CAD build for the part. Positions are in the model's coordinates, mm. A direction names the side the tool comes from. Coordinates: 2 decimals unless noted, no trailing zeros. Order: outer loops, then holes, each group sorted by start corner. A loop starts at its lowest first (then second) coordinate and runs counter-clockwise, first axis right, second up. Notation, with made-up numbers: M 82,86 L 104,86 A14 ccw 104,106 Z; hole C 1,64.25 d3. An arc over 180 degrees is marked long. Write item = value, one per line.
from build123d import *

# Parameters (mm, degrees)
SALIENTE_EXTRUIR1_DEPTH = 3
CROQUIS2_W              = 14
CROQUIS2_H              = 9
CORTAR_EXTRUIR1_DEPTH   = 3
REDONDEO1_R             = 1


with BuildPart() as part:
    # Croquis1 → Saliente-Extruir1 (new body)
    with BuildSketch(Plane.XY):
        Polygon((-32, 29), (-25, 29), (-25, 32), (-15, 32), (-15, 29), (-5, 29), (-5, 32), (5, 32), (5, 29), (15, 29), (15, 32), (25, 32), (25, 29), (32, 29), (32, -29), (25, -29), (25, -32), (15, -32), (15, -29), (5, -29), (5, -32), (-5, -32), (-5, -29), (-15, -29), (-15, -32), (-25, -32), (-25, -29), (-32, -29), align=None)
    extrude(amount=SALIENTE_EXTRUIR1_DEPTH)

    # Croquis2 → Cortar-Extruir1 (cut)
    with BuildSketch(Plane.XY.offset(3)):
        with Locations((0, -13.25)):
            Rectangle(CROQUIS2_W, CROQUIS2_H)
        with Locations((-4.5, 9.5)):
            Rectangle(CROQUIS2_W, CROQUIS2_H)
    extrude(amount=-CORTAR_EXTRUIR1_DEPTH, mode=Mode.SUBTRACT)

    # Redondeo1
    redondeo1_edges = [part.edges().sort_by_distance(p)[0] for p in [
        (7, -8.75, 1.5),
        (7, -17.75, 1.5),
        (-7, -17.75, 1.5),
        (-7, -8.75, 1.5),
        (2.5, 14, 1.5),
        (2.5, 5, 1.5),
        (-11.5, 5, 1.5),
        (-11.5, 14, 1.5),
    ]]
    fillet(redondeo1_edges, radius=REDONDEO1_R)


solid = part.part
(1) Tool access for faces 5 (the face through (-15, -30, 1)), 6 (the face through (-7, -13, 2)), 7 (the face through (-28, -29, 1)): list every direction of +Z, -Z, +X, -X, +Y, -Y with a clear straight run to the whole face (end or side of a thin tool).
Evaluation:
face_5 = +Z, -Z, -Y
face_6 = +Z, -Z
face_7 = +Z, -Z, -X, -Y
(2) Pin check, flat tips, straight feed: pin 1 Ø1.5 at (y, z) = (30, 2) entering from +X; pin 2 Ø5 at (x, y) = (-5, -15.5) entering from -Z; pin 3 Ø1.5 at (x, z) = (-30, 2) entering from +Y. Stop position of each tip, or through.
Evaluation:
pin_1 = 25
pin_2 = 0
pin_3 = 29
(3) Pull direction X, two halves, no side cores. Call faces 1 (the face through (15, 30, 1)), 2 (the face through (-32, 0, 1)), 3 (the face through (0, 32, 1)), 4 (the face through (-10, 29, 1)): +X half, -X half, draft (parallel to the pull), parting line (faces both ways), or undercut.
Evaluation:
face_1 = undercut
face_2 = -X half
face_3 = draft
face_4 = undercut
(4) Wall check: line 1 (Y direction, x = -3.5, z = 1.8); line 2 (X direction, y = -14.5, z = 1.6); line 3 (X direction, y = 6, z = 2.8). Give the ranges that are in metal, low to high. Write a range as from..to.
Evaluation:
line_1 = -32..-17.75, -8.75..5, 14..32
line_2 = -32..-7, 7..32
line_3 = -32..-11.5, 2.5..32
(5) Slice it at C-C, the plane x = 11. Write the cut outline in (y, z), then the cut area to 3 significant figures.
Evaluation:
outline = M -29,0 L 29,0 L 29,3 L -29,3 Z
area = 174 mm²
(6) Slice it at B-B, the plane z = 1.15. State how many separate pieces and enclosed holes the cut face has, then the cut area to 3 significant figures.
Evaluation:
separate_pieces = 1
enclosed_holes = 2
area = 3,640 mm²
(7) Slice it at A-A, the plane y = -14. Write the cut outline in (x, z).
Evaluation:
outline = M -32,0 L -7,0 L -7,3 L -32,3 Z; M 7,0 L 32,0 L 32,3 L 7,3 Z
